CAD build for the part. Positions are in the model's coordinates, mm. Give positions to 0.01 mm unless a question says otherwise; leave off trailing zeros. Order: outer loops, then holes, each group sorted by start corner. A loop starts at its lowest first (then second) coordinate and runs counter-clockwise, first axis right, second up.
Item 1: Flat gauge pins, fed straight in: P1, Ø4, axis at x = 88, z = 185, coming from the -Y side; P2, Ø1.6, axis at y = -1, z = 183.5, coming from the -X side; P3, Ø12, axis at y = -9, z = 186.5, coming from the -X side. Where does each tip first touch, or does it go through?
Item 2: Band-saw the part on A-A on x = 164.5. Give the cut face in (y, z).
Item 3: Wall check: L1, parallel to Y at x = -129, z = 173.75; L2, parallel to Z at x = 17, y = -20.5. Give the ranges that are in metal, low to high.
Item 4: Band-saw the part on C-C on y = -21. Give the cut face in (x, z), plus the area to 3 significant figures.
Item 5: Band-saw the part on B-B on x = -195. Give the cut face in (y, z), plus the area to 3 significant figures.
```python
from build123d import *

# Parameters (mm, degrees)
RESSALTO_EXTRUS_O1_DEPTH = 232
CORTE_EXTRUS_O1_DEPTH    = 50
ESBO_O3_W                = 100
ESBO_O3_H                = 2
CORTE_EXTRUS_O2_DEPTH    = 304.296636974
CORTE_EXTRUS_O3_DEPTH    = 50


with BuildPart() as part:
    # Esboço1 → Ressalto-extrusão1 (new, symmetric)
    with BuildSketch(Plane(origin=(0, 0, 0), x_dir=(0, 0, -1), z_dir=(1, 0, 0))):
        Polygon((-193.7, 0), (-168.3, 0), (-168.3, -2), (-180, -2), (-180, -25.4), (-182, -25.4), (-182, -2), (-193.7, -2), align=None)
    extrude(amount=RESSALTO_EXTRUS_O1_DEPTH, both=True)

    # Esboço2 → Corte-extrusão1 (cut, symmetric)
    with BuildSketch(Plane(origin=(0, 0, 0), x_dir=(1, 0, 0), z_dir=(0, 1, 0))):
        Polygon((-232, -182), (-218.3, -168.3), (-232, -168.3), align=None)
        Polygon((232, -182), (218.3, -168.3), (232, -168.3), align=None)
    extrude(amount=CORTE_EXTRUS_O1_DEPTH, both=True, mode=Mode.SUBTRACT)

    # Esboço3 → Corte-extrusão2 (cut, through all)
    with BuildSketch(Plane(origin=(0, 0, 0), x_dir=(1, 0, 0), z_dir=(0, 1, 0))):
        with Locations((-125, -183)):
            Rectangle(ESBO_O3_W, ESBO_O3_H)
        with Locations((125, -183)):
            Rectangle(ESBO_O3_W, ESBO_O3_H)
    extrude(amount=-CORTE_EXTRUS_O2_DEPTH, mode=Mode.SUBTRACT)

    # Esboço4 → Corte-extrusão3 (cut, symmetric)
    with BuildSketch(Plane(origin=(0, 0, 0), x_dir=(1, 0, 0), z_dir=(0, 1, 0))):
        Polygon((-232, -182), (-220.3, -193.7), (-232, -193.7), align=None)
        Polygon((232, -182), (220.3, -193.7), (232, -193.7), align=None)
    extrude(amount=CORTE_EXTRUS_O3_DEPTH, both=True, mode=Mode.SUBTRACT)


solid = part.part
```
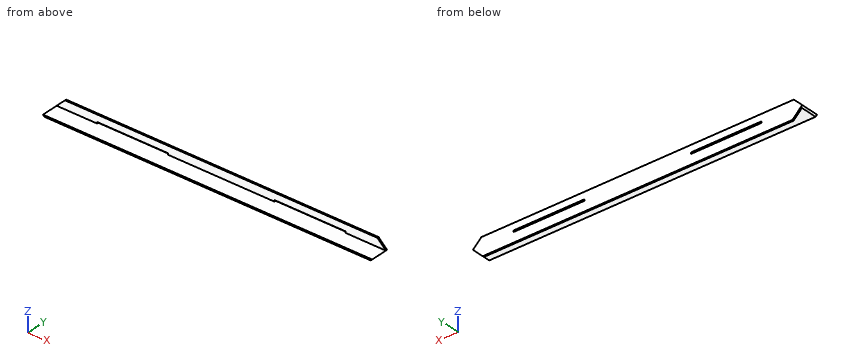
The answers:
1. P1: stops at y = -2
1. P2: stops at x = -231.3
1. P3: stops at x = -232
2. outline: (-25.4, 180) - (-2, 180) - (-2, 168.3) - (0, 168.3) - (0, 182) - (-25.4, 182) - close; (-2, 184) - (0, 184) - (0, 193.7) - (-2, 193.7) - close
3. L1: y = -2 to 0
3. L2: z = 180 to 182
4. outline: (-232, 182) - (-230, 180) - (230, 180) - (232, 182) - close
4. area: 924 mm2
5. outline: (-25.4, 180) - (-2, 180) - (-2, 168.3) - (0, 168.3) - (0, 193.7) - (-2, 193.7) - (-2, 182) - (-25.4, 182) - close
5. area: 97.6 mm2
